Can you work these out from the model? Positions are in its coordinate system, mm. Coordinates: 2 decimals unless noted, no trailing zeros. Loops run counter-clockwise (first coordinate to the right, second up) from the corner with the lowest first, then second, coordinate; pieces in that order, holes last. Notation, with made-up numbers: M -13,-25.75 L 32,-25.75 A10 cw 32,-14.75 Z; hole C -7.75,-32.75 d3. An arc over 180 degrees is marked long. Answer as a JSON object with one key per item and string values. Group by question number.
Item 1: If I drill on line 1 (Z direction, x = 139.5, y = 0.8); line 2 (X direction, y = 2, z = 12); line 3 (Y direction, x = 128.5, z = 6.5) (3 decimals), over which ranges is the centre line in solid material (lowest first)?
Item 2: Suppose I cut it at B-B (y = 9). Write out the boundary of the cut face in (x, z) (3 decimals).
Item 3: Suppose I cut it at A-A (x = 139.5). Write out the boundary of the cut face in (y, z) (1 decimal), then the cut area to 3 significant figures.
Item 4: I'm going to push flat-ended pins straight in: pin 1 Ø1.5 at (x, y) = (102.5, 15.5) entering from +Z (3 decimals); pin 2 Ø3 at (x, z) = (74.5, 14.29) entering from +Y; pin 3 Ø2 at (x, z) = (111, 14) entering from +Y (3 decimals). Where does each tip first touch, or does it pass through?
Item 5: Suppose I cut it at C-C (x = 41). Write out the boundary of the cut face in (y, z) (3 decimals).
Autodesk Inventor part; units mm, degrees
ref_plane "YZ Plane" through (0, 0, 0) normal (1, 0, 0) x (0, 1, 0)
ref_plane "XZ Plane" through (0, 0, 0) normal (0, 1, 0) x (-1, 0, 0)
ref_plane "XY Plane" through (0, 0, 0) normal (0, 0, 1) x (1, 0, 0)
sketch "Sketch1" plane through (0, 0, 0) normal (1, 0, 0) x (0, 1, 0)
  line L0 (0, 0) -> (25.4, 0)
  line L1 (25.4, 0) -> (25.4, 3.175)
  line L2 (25.4, 3.175) -> (0, 3.175)
  line L3 (0, 3.175) -> (0, 0)
  line L4 (0, 0) -> (3.175, 0)
  line L5 (3.175, 0) -> (3.175, 25.4)
  line L6 (3.175, 25.4) -> (0, 25.4)
  line L7 (0, 25.4) -> (0, 0)
  point P0 (3.175, 3.175)
  dimension "d0" = 25.4
  dimension "d1" = 3.175
  dimension "d2" = 3.175
  dimension "d3" = 25.4
extrude "Extrusion1" add sketch "Sketch1" along normal blind 239
sketch "Sketch2" plane through (0, 3.175, 25.4) normal (0, 1, 0) x (1, 0, 0)
  line L0 (0, 22.225) -> (0, 0)
  line L1 (0, 0) -> (239, 0)
  line L2 (239, 22.225) -> (239, 0)
  line L3 (0, 22.225) -> (239, 22.225)
  line L4 (0, 11.1125) -> (74.5, 11.1125)
  line L5 (74.5, 11.1125) -> (139.5, 11.1125)
  circle A0 centre (139.5, 11.1125) radius 2.5
  circle A1 centre (74.5, 11.1125) radius 2.5
  point P0 (0, 25.4)
  dimension "d6" = 74.5
  dimension "d7" = 65
  dimension "d9" = 5
  dimension "d12" = 5
extrude "Extrusion2" cut sketch "Sketch2" against normal blind 10 contours A0 | A1 L5 L4 | L4 L5 A1
properties part number "PERFIL_SOPORTE DEL MOTOR"
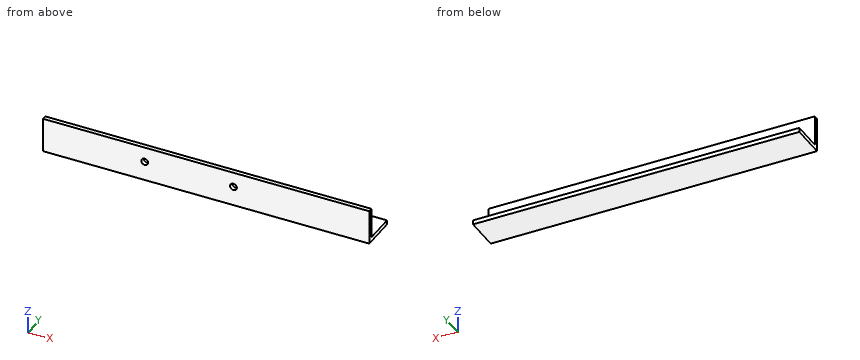
From the geometry:
{
 "1": {"line 1": "0 to 11.79, 16.79 to 25.4", "line 2": "0 to 73.49, 75.51 to 138.49, 140.51 to 239", "line 3": "0 to 3.175"},
 "2": {"outline": "M 0,0 L 239,0 L 239,3.175 L 0,3.175 Z"},
 "3": {"outline": "M 0,0 L 25.4,0 L 25.4,3.2 L 3.2,3.2 L 3.2,11.8 L 0,11.8 Z; M 0,16.8 L 3.2,16.8 L 3.2,25.4 L 0,25.4 Z", "area": "135 mm2"},
 "4": {"pin 1": "z = 3.175", "pin 2": "through", "pin 3": "y = 3.175"},
 "5": {"outline": "M 0,0 L 25.4,0 L 25.4,3.175 L 3.175,3.175 L 3.175,25.4 L 0,25.4 Z"}
}
